```python
from build123d import *

# Parameters (mm, degrees)
SKETCH1_W           = 3.4544
SKETCH1_H           = 12.7
SKETCH1_R           = 1.4732
SKETCH1_W_2         = 15.875
BOSS_EXTRUDE1_DEPTH = 3.175
SKETCH2_W           = 12.7
SKETCH2_H           = 6.35
BOSS_EXTRUDE2_DEPTH = 6.35
SKETCH3_W           = 12.7
SKETCH3_H           = 3.175
BOSS_EXTRUDE3_DEPTH = 3.175
FILLET1_R           = 1.27


with BuildPart() as part:
    # Sketch1 → Boss-Extrude1 (new body)
    # profile 1 of 2: a face of its own
    with BuildSketch(Plane(origin=(0, 0, 0), x_dir=(1, 0, 0), z_dir=(0, 1, 0))):
        with Locations((-9.6647, 0)):
            Rectangle(SKETCH1_W, SKETCH1_H)
        with Locations(Location((-9.6647, -3.81, 0), (0, 0, 270))):
            Circle(SKETCH1_R, mode=Mode.SUBTRACT)
        with Locations(Location((-9.6647, 3.81, 0), (0, 0, 270))):
            Circle(SKETCH1_R, mode=Mode.SUBTRACT)
    # profile 2 of 2: a face of its own
    with BuildSketch(Plane(origin=(0, 0, 0), x_dir=(1, 0, 0), z_dir=(0, 1, 0))):
        Rectangle(SKETCH1_W_2, SKETCH1_H)
    extrude(amount=BOSS_EXTRUDE1_DEPTH)

    # Sketch2 → Boss-Extrude2 (add)
    with BuildSketch(Plane(origin=(7.9375, 0, 0), x_dir=(0, 0, -1), z_dir=(1, 0, 0))):
        with Locations((0, 6.35)):
            Rectangle(SKETCH2_W, SKETCH2_H)
        Polygon((0, 20.523522628), (6.35, 9.525), (-6.35, 9.525), align=None)
    extrude(amount=-BOSS_EXTRUDE2_DEPTH)

    # Sketch3 → Boss-Extrude3 (add)
    with BuildSketch(Plane.ZY.offset(11.3919)):
        with Locations((0, 1.5875)):
            Rectangle(SKETCH3_W, SKETCH3_H)
    extrude(amount=BOSS_EXTRUDE3_DEPTH)

    # Fillet1
    fillet1_edges = [part.edges().sort_by_distance(p)[0] for p in [
        (1.5875, 3.175, 0),
    ]]
    fillet(fillet1_edges, radius=FILLET1_R)


solid = part.part
```
CAD build for the part. Positions are in the model's coordinates, mm. A direction names the side the tool comes from. Coordinates: 2 decimals unless noted, no trailing zeros. Order: outer loops, then holes, each group sorted by start corner. A loop starts at its lowest first (then second) coordinate and runs counter-clockwise, first axis right, second up.
(1) Drill centre lines: L1, parallel to X at y = 1.6, z = 3.81; L2, parallel to Y at x = -12.25, z = -2 (3 decimals); L3, parallel to X at y = 8.25, z = 0.25. Where is each one in solid material? Low to high.
Solution:
L1: x = -14.57 to -11.14, -8.19 to 7.94
L2: y = 0 to 3.175
L3: x = 1.59 to 7.94
(2) Saw through at B-B, the plane y = 5. Write the cut outline in (x, z), and give its area (3 significant figures).
Solution:
outline: (1.59, -6.35) - (7.94, -6.35) - (7.94, 6.35) - (1.59, 6.35) - close
area: 80.6 mm2
(3) Saw through at D-D, the plane y = 10.25. Write the cut outline in (x, z).
Solution:
outline: (1.59, -5.93) - (7.94, -5.93) - (7.94, 5.93) - (1.59, 5.93) - close
(4) Pin check, flat tips, straight feed: pin 1 Ø5 at (x, y) = (1, 10.5) entering from -Z; pin 2 Ø4 at (x, z) = (2.5, -3) entering from +Y; pin 3 Ø8 at (x, y) = (5, 17.5) entering from -Z; pin 4 Ø4 at (y, z) = (11, 1.5) entering from -X. Stop position of each tip, or through.
Solution:
pin 1: stops at z = -6.35
pin 2: stops at y = 18.79
pin 3: stops at z = -4.06
pin 4: stops at x = 1.59
(5) Mould opens along X. For faces 1 (the face through (-1, 3, 6.35)), 2 (the face through (-8.42, 1.57, -3.02)), 3 (the face through (7.938, 8, 0)) say: released by +X, released by -X, zero draft, split by the parting line, or undercut.
Solution:
face 1: zero draft
face 2: undercut
face 3: released by +X
(6) Saw through at C-C, the plane z = 3.81. Write the cut outline in (x, y) (1 decimal), and give its area (3 significant figures).
Solution:
outline: (-14.6, 0) - (-11.1, 0) - (-11.1, 3.2) - (-14.6, 3.2) - close; (-8.2, 0) - (7.9, 0) - (7.9, 13.9) - (1.6, 13.9) - (1.6, 4.4) arc R1.3 cw to (0.3, 3.2) - (-8.2, 3.2) - close
area: 131 mm2
(7) Which spindle directions (+Z, -Z, +X, -X, +Y, -Y) get a long thin tool onto all of the face, cutting with end or side? Do faces 4 (the face through (4.81, 14.95, 3.22)), 5 (the face through (1.588, 11, 0)). Say none if no direction does.
Solution:
face 4: +Z, +X, -X, +Y
face 5: +Z, -Z, -X, +Y
(8) Saw through at A-A, the plane z = -3.5. Write the cut outline in (x, y) (1 decimal).
Solution:
outline: (-14.6, 0) - (-11.1, 0) - (-11.1, 3.2) - (-14.6, 3.2) - close; (-8.2, 0) - (7.9, 0) - (7.9, 14.5) - (1.6, 14.5) - (1.6, 4.4) arc R1.3 cw to (0.3, 3.2) - (-8.2, 3.2) - close
